```python
from build123d import *

# Parameters (mm, degrees)
BOSS_EXTRUDE1_DEPTH = 41.97
SKETCH2_R           = 10.33
CUT_EXTRUDE2_DEPTH  = 1.5
CUT_EXTRUDE2_TAPER  = 45


with BuildPart() as part:
    # Sketch1 → Boss-Extrude1 (new body)
    with BuildSketch(Plane(origin=(0, 0, 0), x_dir=(1, 0, 0), z_dir=(0, 1, 0))):
        Polygon((0, 0), (42.05, 0), (42.05, 41.7), (38.95, 41.7), (38.95, 3.1), (0, 3.1), align=None)
    extrude(amount=BOSS_EXTRUDE1_DEPTH)

    # Sketch2 → Cut-Extrude2 (cut)
    with BuildSketch(Plane(origin=(42.05, 0, 0), x_dir=(-1, 0, 0), z_dir=(0, 0, -1))):
        with Locations((24.17, 20.985)):
            Circle(SKETCH2_R)
    extrude(amount=CUT_EXTRUDE2_DEPTH, taper=CUT_EXTRUDE2_TAPER, mode=Mode.SUBTRACT)


solid = part.part
```
Input: part model. Units: mm. Frame: model coordinates. A direction names the side the tool comes from. Round coordinates to 2 decimals unless told otherwise and drop trailing zeros. Loops run counter-clockwise (first coordinate to the right, second up) from the corner with the lowest first, then second, coordinate; pieces in that order, holes last. Notation, with made-up numbers: M 21,2 L 49,2 A27 cw 49,34 Z; hole C 45,-26.75 d3. An arc over 180 degrees is marked long. Answer in a Markdown table with one row per item. Add a question column.
1. Section D-D (x = 3). Output: boundary loops of the cut face in (y, z), and give its area (3 significant figures).
2. Section A-A (y = 5.5). Output: boundary loops of the cut face in (x, z), and give its area (3 significant figures).
3. Section C-C (z = -38.5). Output: boundary loops of the cut face in (x, y).
4. Ray query, probe 1 along Z at (x, y) = (18, 18.5); probe 2 along X at (y, z) = (6.5, -8); probe 3 along Z at (x, y) = (36, 27). Return the intervals inside material, ascending.
5. Section B-B (x = 17.88). Output: boundary loops of the cut face in (y, z) (3 decimals), and give its area (3 significant figures).
6. Mould query, pull axis Y, two halves, no side actions, for faces 1 (the face through (38.95, 21, -23)), 2 (the face through (30, 41.97, -2)), 3 (the face through (30, 0, -2)), 4 (the face through (18, 21, -1.5)). Classes: released by +Y, released by -Y, zero draft, split by the parting line, or undercut.
7. Contact query for flat-ended pins moving along their axis: pin 1 (9 mm diameter, centred on x = 22, y = 20.5, fed in from +Z); pin 2 (5 mm diameter, centred on y = 11.5, z = -31, fed in from -X); pin 3 (6 mm diameter, centred on x = 27, y = 15, fed in from -Z). Output: stop coordinate, or through.
8. Set-up query: faces 5 (the face through (0, 21, -2)), 6 (the face through (20, 21, -3.1)). Return all of +Z, -Z, +X, -X, +Y, -Y with unobstructed straight access to the full face (end or side cutting, diameter ignored); none if empty.
Values follow:
| question | item | result |
|---|---|---|
| 1 | outline | M 0,-3.1 L 41.97,-3.1 L 41.97,0 L 0,0 Z |
| 1 | area | 130 mm^2 |
| 2 | outline | M 0,-3.1 L 38.95,-3.1 L 38.95,-41.7 L 42.05,-41.7 L 42.05,0 L 0,0 Z |
| 2 | area | 250 mm^2 |
| 3 | outline | M 38.95,0 L 42.05,0 L 42.05,41.97 L 38.95,41.97 Z |
| 4 | probe 1 | -3.1 to -1.5 |
| 4 | probe 2 | 38.95 to 42.05 |
| 4 | probe 3 | -3.1 to 0 |
| 5 | outline | M 0,-3.1 L 41.97,-3.1 L 41.97,0 L 31.315,0 L 29.815,-1.5 L 12.155,-1.5 L 10.655,0 L 0,0 Z |
| 5 | area | 101 mm^2 |
| 6 | face 1 | zero draft |
| 6 | face 2 | released by +Y |
| 6 | face 3 | released by -Y |
| 6 | face 4 | undercut |
| 7 | pin 1 | z = -1.5 |
| 7 | pin 2 | x = 38.95 |
| 7 | pin 3 | z = -3.1 |
| 8 | face 5 | +Z, -Z, -X, +Y, -Y |
| 8 | face 6 | -Z, -X, +Y, -Y |
